```python
from build123d import *

# Parameters (mm, degrees)
SKETCH_1_W          = 111
SKETCH_1_H          = 61
SKETCH_1_W_2        = 107
SKETCH_1_H_2        = 57
EXTRUDE_1_DEPTH     = 10
SKETCH_3_W          = 111
SKETCH_3_H          = 61
EXTRUDE_1_2_DEPTH   = 2
SKETCH_5_W          = 27.999833333
SKETCH_5_H          = 10.1
EXTRUDE_2_DEPTH     = 8
EXTRUDE_3_REACH     = 127.104
SKETCH_6_W          = 107
SKETCH_6_H          = 57
SKETCH_6_W_2        = 101
SKETCH_6_H_2        = 51
EXTRUDE_4_REACH     = 126.165
SKETCH_8_W          = 6
SKETCH_8_H          = 10.1
CUT_EXTRUDE_1_DEPTH = 10
SKETCH_9_W          = 3
SKETCH_9_H          = 10.1
EXTRUDE_7_DEPTH     = 8


with BuildPart() as part:
    # 草圖1 → Extrude 1 (new body)
    with BuildSketch(Plane(origin=(0, 0, 0), x_dir=(1, 0, 0), z_dir=(0, 1, 0))):
        with Locations((53.5, 28.5)):
            Rectangle(SKETCH_1_W, SKETCH_1_H)
        with Locations((53.5, 28.5)):
            Rectangle(SKETCH_1_W_2, SKETCH_1_H_2, mode=Mode.SUBTRACT)
    extrude(amount=-EXTRUDE_1_DEPTH)

    # 草圖3 → Extrude 1 2 (add)
    with BuildSketch(Plane(origin=(0, -10, 0), x_dir=(-1, 0, 0), z_dir=(0, -1, 0))):
        with Locations((-53.5, 28.5)):
            Rectangle(SKETCH_3_W, SKETCH_3_H)
    extrude(amount=EXTRUDE_1_2_DEPTH)

    # 草圖5 → 填料-伸長2 (add)
    with BuildSketch(Plane.XZ.offset(12)):
        Polygon((-2, -23.5), (-2, -33.5), (-2, -43.5), (37.999833333, -43.5), (37.999833333, -13.5), (-2, -13.5), align=None)
        with Locations((13.999916667, -28.45)):
            Rectangle(SKETCH_5_W, SKETCH_5_H, mode=Mode.SUBTRACT)
    extrude(amount=EXTRUDE_2_DEPTH)

    # 草圖6 → 填料-伸長3 (add, up to next)
    with BuildSketch(Plane(origin=(0, -3, 0), x_dir=(1, 0, 0), z_dir=(0, 1, 0)), mode=Mode.PRIVATE) as extrude_3_sk1:
        with Locations((53.5, 28.5)):
            Rectangle(SKETCH_6_W, SKETCH_6_H)
        with Locations((53.5, 28.5)):
            Rectangle(SKETCH_6_W_2, SKETCH_6_H_2, mode=Mode.SUBTRACT)
    extrude_3_tool1 = extrude(extrude_3_sk1.sketch, amount=-EXTRUDE_3_REACH, mode=Mode.PRIVATE) - part.part
    add(extrude_3_tool1.solids().sort_by_distance((105.787647, -3, -28.5))[0])

    # 草圖7 → 填料-伸長4 (add, up to next)
    with BuildSketch(Plane(origin=(0, 0, -3), x_dir=(-1, 0, 0), z_dir=(0, 0, -1)), mode=Mode.PRIVATE) as extrude_4_sk1:
        Polygon((-104, -3), (-3, -10), (-104, -10), align=None)
    extrude_4_tool1 = extrude(extrude_4_sk1.sketch, amount=EXTRUDE_4_REACH, mode=Mode.PRIVATE) - part.part
    add(extrude_4_tool1.solids().sort_by_distance((70.333333, -7.666667, -3))[0])

    # 草圖8 → 除料-伸長1 (cut)
    with BuildSketch(Plane.XZ.offset(12)):
        with Locations((6, -28.45)):
            Rectangle(SKETCH_8_W, SKETCH_8_H)
    extrude(amount=-CUT_EXTRUDE_1_DEPTH, mode=Mode.SUBTRACT)

    # 草圖9 → 填料-伸長7 (add)
    with BuildSketch(Plane.XZ.offset(12)):
        with Locations((1.5, -28.45)):
            Rectangle(SKETCH_9_W, SKETCH_9_H)
    extrude(amount=EXTRUDE_7_DEPTH)


solid = part.part
```
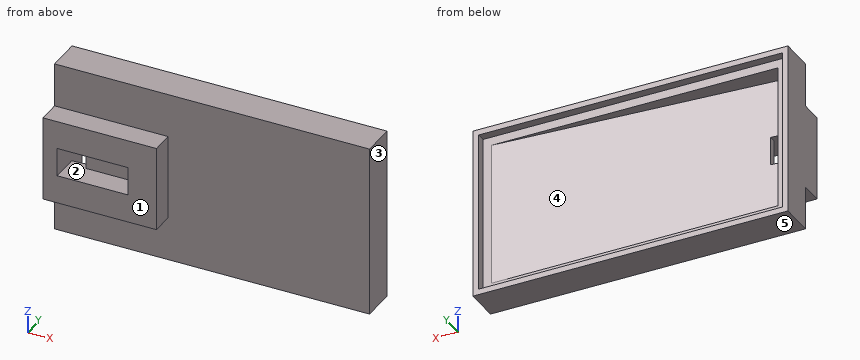
Input: part model. Units: mm. Frame: model coordinates. Face numbers are marked on the shaded views. A direction names the side the tool comes from. Round coordinates to 2 decimals unless told otherwise and drop trailing zeros. Loops run counter-clockwise (first coordinate to the right, second up) from the corner with the lowest first, then second, coordinate; pieces in that order, holes last.
1) Section query C-C on x = 6. Return the cut outline in (y, z), plus the area to 3 significant figures.
Ans:
outline: (-20, -43.5) - (-12, -43.5) - (-12, -59) - (0, -59) - (0, -57) - (-3, -57) - (-3, -54) - (-9.79, -54) - (-9.79, -33.5) - (-20, -33.5) - close; (-20, -23.4) - (-9.79, -23.4) - (-9.79, -3) - (-3, -3) - (-3, 0) - (0, 0) - (0, 2) - (-12, 2) - (-12, -13.5) - (-20, -13.5) - close
area: 352 mm2
2) Section query A-A on y = -14.25. Return the cut outline in (x, z), plus the area to 3 significant figures.
Ans:
outline: (-2, -43.5) - (38, -43.5) - (38, -13.5) - (-2, -13.5) - close; hole (3, -33.5) - (28, -33.5) - (28, -23.4) - (3, -23.4) - close
area: 947 mm2
3) Pull-direction query (Z, two-part tool) for the marked faces 3, 4 and 5; classes: released by +Z, released by -Z, zero draft, split by the parting line, or undercut.
Ans:
face 3: zero draft
face 4: undercut
face 5: released by -Z
4) Section query B-B on z = -51.5. Return the cut outline in (x, y), plus the area to 4 significant figures.
Ans:
outline: (-2, -12) - (109, -12) - (109, 0) - (107, 0) - (107, -3) - (104, -3) - (3, -10) - (3, -3) - (0, -3) - (0, 0) - (-2, 0) - close
area: 657.5 mm2
5) Pin query (flat end, axial travel): pin 1 (2.5 mm diameter, centred on x = 13, y = -14.5, fed in from -Z); pin 2 (2 mm diameter, centred on x = 57, z = -49.5, fed in from +Y); pin 3 (10 mm diameter, centred on x = 50.5, z = -14.5, fed in from +Y). Return the tip coordinate at first contact, or that it passes through.
Ans:
pin 1: stops at z = -43.5
pin 2: stops at y = -6.19
pin 3: stops at y = -6.36
6) Set-up query: the marked faces 1 and 2. Return all of +Z, -Z, +X, -X, +Y, -Y with unobstructed straight access to the full face (end or side cutting, diameter ignored); none if empty.
Ans:
face 1: +Z, -Z, +X, -X, -Y
face 2: -Y
7) Material intervals for line 1 (Z direction, x = 52.5, y = -4); line 2 (X direction, y = -16, z = -29.5); line 3 (X direction, y = -2.5, z = -25.5), sorted ascending.
Ans:
line 1: z = -59 to -54, -3 to 2
line 2: x = -2 to 3, 28 to 38
line 3: x = -2 to 0, 107 to 109
8) Section query D-D on x = 32. Return the cut outline in (y, z).
Ans:
outline: (-20, -43.5) - (-12, -43.5) - (-12, -59) - (0, -59) - (0, -57) - (-3, -57) - (-3, -54) - (-7.99, -54) - (-7.99, -3) - (-3, -3) - (-3, 0) - (0, 0) - (0, 2) - (-12, 2) - (-12, -13.5) - (-20, -13.5) - close
